```python
from build123d import *

# Parameters (mm, degrees)
BOSS_EXTRUDE1_DEPTH                 = 22.479
F_5_32_0_15625_DIAMETER_HOLE1_D     = 3.96875
F_5_32_0_15625_DIAMETER_HOLE1_DEPTH = 31.75
SKETCH17_R                          = 14.097
CUT_EXTRUDE1_DEPTH                  = 1
CUT_EXTRUDE1_DEPTH_BACK             = 45.958
BOSS_EXTRUDE2_DEPTH                 = 19.05
BOSS_EXTRUDE3_DEPTH                 = 16.256


with BuildPart() as part:
    # Sketch2 → Boss-Extrude1 (new body, symmetric)
    with BuildSketch(Plane.XY):
        Polygon((22.06839298, 16.2941), (10.63839298, 16.2941), (9.525, 15.4559), (-9.525, 15.4559), (-10.63839298, 16.2941), (-22.06839298, 16.2941), (-22.3012, 15.619179923), (-22.3012, 7.4803), (-20.955, 6.1341), (-20.955, -15.4559), (20.955, -15.4559), (20.955, 6.1341), (22.3012, 7.4803), (22.3012, 15.619179923), align=None)
    extrude(amount=BOSS_EXTRUDE1_DEPTH, both=True)

    # 5/32 (0.15625) Diameter Hole1
    with Locations(Plane(origin=(0, 16.2941, 0), x_dir=(1, 0, 0), z_dir=(0, 1, 0))):
        with Locations((-16.35339298, 14.859), (-16.35339298, -14.859), (16.35339298, -14.859), (16.35339298, 14.859)):
            Hole(F_5_32_0_15625_DIAMETER_HOLE1_D / 2, depth=F_5_32_0_15625_DIAMETER_HOLE1_DEPTH)

    # Sketch17 → Cut-Extrude1 (cut, two sides)
    with BuildSketch(Plane.XY.offset(22.479)) as cut_extrude1_sk:
        with Locations((0, -3.7211)):
            Circle(SKETCH17_R)
    extrude(amount=CUT_EXTRUDE1_DEPTH, mode=Mode.SUBTRACT)
    extrude(cut_extrude1_sk.sketch, amount=-CUT_EXTRUDE1_DEPTH_BACK, mode=Mode.SUBTRACT)

    # Sketch18 → Boss-Extrude2 (add, symmetric)
    with BuildSketch(Plane.XY):
        with BuildLine():
            Line((-7.811522128, -15.4559), (-7.037407323, -14.292991892))
            ThreePointArc((-7.037407323, -14.292991892), (0, 8.9789), (7.037407323, -14.292991892))
            Line((7.037407323, -14.292991892), (7.811522128, -15.4559))
            ThreePointArc((7.811522128, -15.4559), (0, 10.3759), (-7.811522128, -15.4559))
        make_face()
    extrude(amount=BOSS_EXTRUDE2_DEPTH, both=True)

    # Sketch19 → Boss-Extrude3 (add, symmetric)
    with BuildSketch(Plane.XY):
        with BuildLine():
            Line((-7.037407323, -14.292991892), (-4.539127723, -10.53997027))
            ThreePointArc((-4.539127723, -10.53997027), (0, 4.4704), (4.539127723, -10.53997027))
            Line((4.539127723, -10.53997027), (7.037407323, -14.292991892))
            ThreePointArc((7.037407323, -14.292991892), (0, 8.9789), (-7.037407323, -14.292991892))
        make_face()
    extrude(amount=BOSS_EXTRUDE3_DEPTH, both=True)


solid = part.part
```
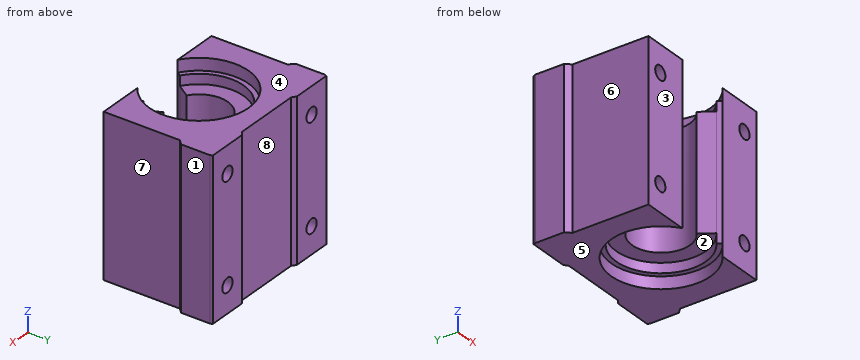
Read the model definition and answer for the solid it produces. Units are mm, in the model's axes. Face numbers are marked on the shaded views. A direction names the side the tool comes from. Give positions to 0.01 mm unless a question says otherwise; leave off trailing zeros. Write each loop counter-clockwise with the first axis right and the second up, starting at its lowest first coordinate (ties: lowest second). Pieces come first, ordered by that corner, then holes. Notation, with made-up numbers: M 78.25,-31 L 122.25,-31 A6 cw 122.25,-23 Z; hole C 5.5,-5 d2. An arc over 180 degrees is marked long. Put each result on its own line as item: value. Start each with the question number.
1. For a pull along X with two mould halves and no side action, classify the marked faces 1, 2 and 3 as released by +X, released by -X, zero draft, split by the parting line, or undercut.
2. Which of the six approach directions +Z, -Z, +X, -X, +Y, -Y give full straight-line access (tool end or side, diameter ignored) to the marked faces 4, 5, 6, 7 and 8?
3. Consider line 1 along X through (y, z) = (10, -14); line 2 along X through (y, z) = (2.5, 15.5) (3 decimals); line 3 along Z through (x, y) = (15.5, -9). Determine where each line is inside the solid, lowest interval first.
4. Each of these flat-tipped pins is pushed along its axis until it touches: pin 1 Ø4 at (x, z) = (-1.5, 6.5) entering from +Y; pin 2 Ø3.5 at (x, z) = (16.35, 14.86) entering from -Y; pin 3 Ø3 at (y, z) = (5.5, 3) entering from +X; pin 4 Ø6 at (y, z) = (-1.5, 5) entering from +X (3 decimals). Where does it stop, or does it pass through?
5. The part is cut by section B-B, the plane z = 12. Give the vertices of the cut face in (x, y) (1 decimal), and give its area (3 significant figures).
6. The part is cut by section A-A, the plane x = 0. Give the vertices of the cut face in (y, z), and give its area (3 significant figures).
7. The part is cut by section C-C, the plane x = 15.5. Give the vertices of the cut face in (y, z).
Final values:
1. face 1: released by +X
1. face 2: undercut
1. face 3: zero draft
2. face 4: +Z, +X, -X, +Y, -Y
2. face 5: -Z, +X, -X, +Y, -Y
2. face 6: +Z, -Z, -X, -Y
2. face 7: +Z, -Z, +X, -Y
2. face 8: +Z, -Z, +Y
3. line 1: x = -22.3 to -18.14, -14.56 to 14.56, 18.14 to 22.3
3. line 2: x = -20.955 to -18.231, -14.475 to -5.329, 5.329 to 14.475, 18.231 to 20.955
3. line 3: z = -22.48 to -16.65, -13.07 to 13.07, 16.65 to 22.48
4. pin 1: stops at y = 15.46
4. pin 2: passes through
4. pin 3: stops at x = 21.82
4. pin 4: stops at x = 20.955
5. outline: M -22.3,7.5 L -21,6.1 L -21,-15.5 L -7.8,-15.5 L -4.5,-10.5 A8.2 cw long 4.5,-10.5 L 7.8,-15.5 L 21,-15.5 L 21,6.1 L 22.3,7.5 L 22.3,15.6 L 22.1,16.3 L 10.6,16.3 L 9.5,15.5 L -9.5,15.5 L -10.6,16.3 L -22.1,16.3 L -22.3,15.6 Z
5. area: 1,080 mm²
6. outline: M 4.47,-16.26 L 8.98,-16.26 L 8.98,-19.05 L 10.38,-19.05 L 10.38,-22.48 L 15.46,-22.48 L 15.46,22.48 L 10.38,22.48 L 10.38,19.05 L 8.98,19.05 L 8.98,16.26 L 4.47,16.26 Z
6. area: 428 mm²
7. outline: M -15.46,-22.48 L 16.29,-22.48 L 16.29,-16.65 L -15.46,-16.65 Z; M -15.46,-13.07 L 16.29,-13.07 L 16.29,13.07 L -15.46,13.07 Z; M -15.46,16.65 L 16.29,16.65 L 16.29,22.48 L -15.46,22.48 Z
